Can you work these out from the model? Positions are in its coordinate system, mm. Give positions to 0.01 mm unless a question says otherwise; leave off trailing zeros. Order: outer loops, then holes, each group sorted by start corner. A loop starts at its lowest first (then second) coordinate and runs counter-clockwise, first axis right, second up. Notation, with made-up numbers: (47.25, 23) - (67.25, 23) arc R22 cw to (67.25, 44) - close; hole circle Ø8 at (17.5, 3.5). An arc over 180 degrees is marked (long way). One line per question, with ' | ' between items.
```python
from build123d import *

# Parameters (mm, degrees)
F0_W     = 50.8
F0_H     = 50.8
F1_DEPTH = 9.525
F2_DEPTH = 3.175
F3_R     = 5.08


with BuildPart() as f1:
    # F0 (on Top) → F1 (new body)
    with BuildSketch(Plane.XY):
        Rectangle(F0_W, F0_H)
        with BuildLine():
            ThreePointArc((12.941801, 18.843816), (15.972171, 20.351047), (19.127946, 19.127946))
            ThreePointArc((19.127946, 19.127946), (20.03644, 17.768287), (20.355461, 16.164461))
            ThreePointArc((20.355461, 16.164461), (19.958776, 14.384671), (18.843816, 12.941801))
            ThreePointArc((18.843816, 12.941801), (21.832879, 6.775322), (22.86, 0))
            ThreePointArc((22.86, 0), (21.832879, -6.775322), (18.843816, -12.941801))
            ThreePointArc((18.843816, -12.941801), (19.958776, -14.384671), (20.355461, -16.164461))
            ThreePointArc((20.355461, -16.164461), (17.588945, -20.105949), (12.941801, -18.843816))
            ThreePointArc((12.941801, -18.843816), (0, -22.86), (-12.941801, -18.843816))
            ThreePointArc((-12.941801, -18.843816), (-19.127946, -19.127946), (-18.843816, -12.941801))
            ThreePointArc((-18.843816, -12.941801), (-22.86, 0), (-18.843816, 12.941801))
            ThreePointArc((-18.843816, 12.941801), (-19.127946, 19.127946), (-12.941801, 18.843816))
            ThreePointArc((-12.941801, 18.843816), (0, 22.86), (12.941801, 18.843816))
        make_face(mode=Mode.SUBTRACT)
        with BuildLine():
            ThreePointArc((13.200976, 13.200976), (11.977875, 15.972171), (12.941801, 18.843816))
            ThreePointArc((12.941801, 18.843816), (0, 22.86), (-12.941801, 18.843816))
            ThreePointArc((-12.941801, 18.843816), (-12.222973, 17.588945), (-11.973461, 16.164461))
            ThreePointArc((-11.973461, 16.164461), (-14.384671, 12.370146), (-18.843816, 12.941801))
            ThreePointArc((-18.843816, 12.941801), (-22.86, 0), (-18.843816, -12.941801))
            ThreePointArc((-18.843816, -12.941801), (-14.384671, -12.370146), (-11.973461, -16.164461))
            ThreePointArc((-11.973461, -16.164461), (-12.222973, -17.588945), (-12.941801, -18.843816))
            ThreePointArc((-12.941801, -18.843816), (0, -22.86), (12.941801, -18.843816))
            ThreePointArc((12.941801, -18.843816), (13.200976, -13.200976), (18.843816, -12.941801))
            ThreePointArc((18.843816, -12.941801), (21.832879, -6.775322), (22.86, 0))
            ThreePointArc((22.86, 0), (21.832879, 6.775322), (18.843816, 12.941801))
            ThreePointArc((18.843816, 12.941801), (15.972171, 11.977875), (13.200976, 13.200976))
        make_face()
        with BuildLine():
            ThreePointArc((15.24, 0), (-14.079924, -5.832096), (10.776307, 10.776307))
            ThreePointArc((10.776307, 10.776307), (14.079924, 5.832096), (15.24, 0))
        make_face(mode=Mode.SUBTRACT)
        with BuildLine():
            ThreePointArc((15.24, 0), (14.079924, 5.832096), (10.776307, 10.776307))
            ThreePointArc((10.776307, 10.776307), (-14.079924, -5.832096), (15.24, 0))
        make_face()
        with BuildLine():
            ThreePointArc((5.588, 0), (-5.162639, -2.138435), (3.951313, 3.951313))
            ThreePointArc((3.951313, 3.951313), (5.162639, 2.138435), (5.588, 0))
        make_face(mode=Mode.SUBTRACT)
    extrude(amount=-F1_DEPTH)

    # F0 (on Top) → F2 (cut)
    with BuildSketch(Plane.XY):
        with BuildLine():
            ThreePointArc((15.24, 0), (14.079924, 5.832096), (10.776307, 10.776307))
            ThreePointArc((10.776307, 10.776307), (-14.079924, -5.832096), (15.24, 0))
        make_face()
        with BuildLine():
            ThreePointArc((5.588, 0), (-5.162639, -2.138435), (3.951313, 3.951313))
            ThreePointArc((3.951313, 3.951313), (5.162639, 2.138435), (5.588, 0))
        make_face(mode=Mode.SUBTRACT)
    extrude(amount=-F2_DEPTH, mode=Mode.SUBTRACT)

    # F3
    f3_edges = [f1.edges().sort_by_distance(p)[0] for p in [
        (-25.4, -25.4, -4.7625),
        (25.4, -25.4, -4.7625),
        (25.4, 25.4, -4.7625),
        (-25.4, 25.4, -4.7625),
    ]]
    fillet(f3_edges, radius=F3_R)


solid = f1.part
```
(1) Will this pin go through, and if not, where does the flat tip stop? pin 1 (3 mm diameter, centred on x = 8, y = -1, fed in from +Z) (3 decimals).
Answer below:
pin 1: z = -3.175
(2) Imagine slicing it at D-D (y = -19.5). List the corners of the cut face in (x, z) for me (3 decimals).
Answer below:
outline: (-25.4, -9.525) - (-18.702, -9.525) - (-18.702, 0) - (-25.4, 0) - close; (-13.627, -9.525) - (13.627, -9.525) - (13.627, 0) - (-13.627, 0) - close; (18.702, -9.525) - (25.4, -9.525) - (25.4, 0) - (18.702, 0) - close
(3) Imagine slicing it at C-C (y = -3). List the corners of the cut face in (x, z) for me (3 decimals), and give its area (3 significant figures).
Answer below:
outline: (-25.4, -9.525) - (-4.714, -9.525) - (-4.714, -3.175) - (-14.942, -3.175) - (-14.942, 0) - (-25.4, 0) - close; (4.714, -9.525) - (25.4, -9.525) - (25.4, 0) - (14.942, 0) - (14.942, -3.175) - (4.714, -3.175) - close | area: 329 mm^2
(4) Imagine slicing it at B-B (z = -7.5). List the corners of the cut face in (x, y) for me, and give its area (3 significant figures).
Answer below:
outline: (-25.4, -20.32) arc R5.08 ccw to (-20.32, -25.4) - (20.32, -25.4) arc R5.08 ccw to (25.4, -20.32) - (25.4, 20.32) arc R5.08 ccw to (20.32, 25.4) - (-20.32, 25.4) arc R5.08 ccw to (-25.4, 20.32) - close; hole (-12.94, -18.84) arc R4.19 ccw to (-11.97, -16.16) arc R4.19 ccw (long way) to start; hole (-12.94, 18.84) arc R4.19 ccw (long way) to (-11.97, 16.16) arc R4.19 ccw to start; hole circle Ø11.18 at (0, 0); hole (12.94, 18.84) arc R4.19 ccw to (13.2, 13.2) arc R4.19 ccw to (18.84, 12.94) arc R4.19 ccw to (20.36, 16.16) arc R4.19 ccw to (19.13, 19.13) arc R4.19 ccw to start; hole (18.84, -12.94) arc R4.19 ccw (long way) to (20.36, -16.16) arc R4.19 ccw to start | area: 2,240 mm^2
(5) If we mould it in two halves opening along X, with no side actions, what happens to faces 1 (the face through (-23.951, 23.872, -4.829)), 2 (the face through (0, -25.4, -5)), 3 (the face through (0, -7, -3.175))? For each: released by +X, released by -X, zero draft, split by the parting line, or undercut.
Answer below:
face 1: released by -X | face 2: zero draft | face 3: undercut
(6) If I drill on line 1 (Y direction, x = -16, z = -7.25); line 2 (Y direction, x = 19, z = -4.25); line 3 (Y direction, x = -13, z = -0.25), over which ranges is the centre line in solid material (lowest first)?
Answer below:
line 1: -25.4 to -20.35, -11.98 to 11.98, 20.35 to 25.4 | line 2: -25.4 to -19.25, -13.08 to 13.08, 19.25 to 25.4 | line 3: -25.4 to -18.91, -13.42 to -7.95, 7.95 to 13.42, 18.91 to 25.4
(7) Imagine slicing it at A-A (x = 0). List the corners of the cut face in (y, z) for me (3 decimals), and give its area (3 significant figures).
Answer below:
outline: (-25.4, -9.525) - (-5.588, -9.525) - (-5.588, -3.175) - (-15.24, -3.175) - (-15.24, 0) - (-25.4, 0) - close; (5.588, -9.525) - (25.4, -9.525) - (25.4, 0) - (15.24, 0) - (15.24, -3.175) - (5.588, -3.175) - close | area: 316 mm^2
